Input: part model. Units: mm. Frame: model coordinates. Give positions to 0.01 mm unless a question says otherwise; leave off trailing zeros. Loops run counter-clockwise (first coordinate to the right, second up) from the corner with the lowest first, then second, coordinate; pieces in that order, holes last. Notation, with made-up numbers: (-29.75, 18.25) - (-11.75, 18.25) arc R7 cw to (-11.75, 26.25) - close; hole circle Ø3 at (-4, -11.75). An arc over 180 degrees is marked (long way). One line per item, written item: value.
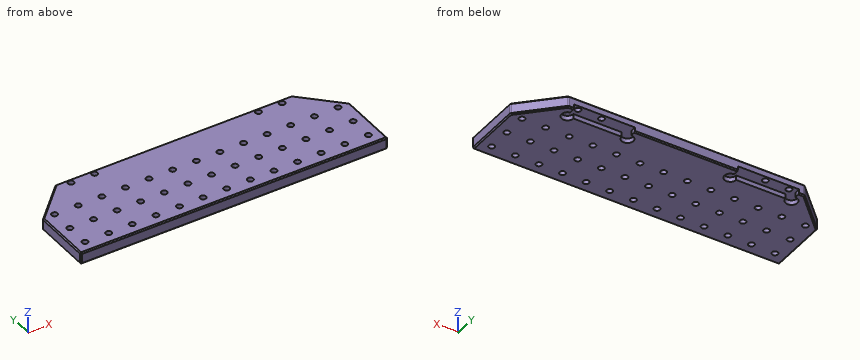
from build123d import *

# Parameters (mm, degrees)
EXTRUDE_1_DEPTH             = 3
EXTRUDE_1_DEPTH_BACK        = 2
SKETCH_2_W                  = 130
SKETCH_2_H                  = 40
SKETCH_6_W                  = 25.903315895
SKETCH_6_H                  = 5
CUT_EXTRUDE_6_DEPTH         = 2
SKETCH_7_R                  = 2.5
CUT_EXTRUDE_7_DEPTH         = 2
CHAMFER_1_SIZE              = 15
M3X0_5_1_D                  = 2.5
M3X0_5_1_DEPTH              = 8.5
M3X0_5_1_TIP                = 0.751075774
FILLET_1_R                  = 1
PATTERN_LINEAR_1_COUNT      = 7
PATTERN_LINEAR_1_PITCH      = 10
PATTERN_LINEAR_1_COUNT_DIR2 = 3
PATTERN_LINEAR_1_PITCH_DIR2 = 10
PATTERN_LINEAR_2_COUNT      = 7
PATTERN_LINEAR_2_PITCH      = 10
PATTERN_LINEAR_2_COUNT_DIR2 = 3
PATTERN_LINEAR_2_PITCH_DIR2 = 10
CHAMFER_2_SIZE              = 0.5


with BuildPart() as part:
    # ｽｹｯﾁ2 → ﾎﾞｽ - 押し出し1 (new, two sides: drawn at the far end of the back side and taken through both)
    with BuildSketch(Plane.XY.offset(-EXTRUDE_1_DEPTH_BACK)):
        with Locations((-80.49999999, -32)):
            Rectangle(SKETCH_2_W, SKETCH_2_H)
    extrude(amount=EXTRUDE_1_DEPTH + EXTRUDE_1_DEPTH_BACK)

    # ｽｹｯﾁ6 → ｶｯﾄ - 押し出し6 (cut)
    with BuildSketch(Plane(origin=(0, 0, -2), x_dir=(-1, 0, 0), z_dir=(0, 0, -1))):
        with Locations((115.230241042, -14.5)):
            Rectangle(SKETCH_6_W, SKETCH_6_H)
        with Locations((45.76975894, -14.5)):
            Rectangle(SKETCH_6_W, SKETCH_6_H)
    extrude(amount=-CUT_EXTRUDE_6_DEPTH, mode=Mode.SUBTRACT)

    # ｽｹｯﾁ7 → ｶｯﾄ - 押し出し7 (cut)
    with BuildSketch(Plane(origin=(0, 0, -2), x_dir=(-1, 0, 0), z_dir=(0, 0, -1))):
        with Locations((33.318100992, -17)):
            Circle(SKETCH_7_R)
        with Locations((128.181898989, -17)):
            Circle(SKETCH_7_R)
        with Locations((102.278583094, -17)):
            Circle(SKETCH_7_R)
        with Locations((58.721416887, -17)):
            Circle(SKETCH_7_R)
    extrude(amount=-CUT_EXTRUDE_7_DEPTH, mode=Mode.SUBTRACT)

    # 面取り1
    chamfer_1_edges = [part.edges().sort_by_distance(p)[0] for p in [
        (-145.49999999, -12, 0.5),
        (-15.49999999, -12, 0.5),
    ]]
    chamfer(chamfer_1_edges, length=CHAMFER_1_SIZE)

    # M3x0.5 ねじ穴1
    with Locations(Plane(origin=(0, 0, 0), x_dir=(-1, 0, 0), z_dir=(0, 0, -1))):
        with Locations((35.818100992, -14), (125.181898989, -14), (45.818100992, -14), (115.181898989, -14)):
            Hole(M3X0_5_1_D / 2, depth=M3X0_5_1_DEPTH)
            with Locations((0, 0, -(M3X0_5_1_DEPTH + M3X0_5_1_TIP / 2))):  # 118° drill point
                Cone(0, M3X0_5_1_D / 2, M3X0_5_1_TIP, mode=Mode.SUBTRACT)

    # ﾌｨﾚｯﾄ1
    fillet_1_edges = [part.edges().sort_by_distance(p)[0] for p in [
        (-30.49999999, -12, 0.5),
        (-130.49999999, -12, 0.5),
        (-145.49999999, -27, 0.5),
        (-15.49999999, -27, 0.5),
    ]]
    fillet(fillet_1_edges, radius=FILLET_1_R)

    # ｽｹｯﾁ11 → M3x0.5 ねじ穴2 (revolve, cut)
    with BuildSketch(Plane(origin=(-80.49999999, -47, -2), x_dir=(0, 1, 0), z_dir=(1, 0, 0))):
        Polygon((0, 0), (0, 9.251075774), (1.25, 8.5), (1.25, 0), align=None)
    m3x0_5_2 = revolve(axis=Axis((-80.49999999, -47, -8.35), (0, 0, 1)), mode=Mode.SUBTRACT)

    # 直線ﾊﾟﾀｰﾝ1: M3x0.5 _2 7 × 3
    with Locations(*[(i * PATTERN_LINEAR_1_PITCH, j * PATTERN_LINEAR_1_PITCH_DIR2, 0) for i in range(PATTERN_LINEAR_1_COUNT) for j in range(PATTERN_LINEAR_1_COUNT_DIR2) if (i, j) != (0, 0)]):
        add(m3x0_5_2, mode=Mode.SUBTRACT)

    # 直線ﾊﾟﾀｰﾝ2: M3x0.5 _2 7 × 3
    with Locations(*[(-i * PATTERN_LINEAR_2_PITCH, j * PATTERN_LINEAR_2_PITCH_DIR2, 0) for i in range(PATTERN_LINEAR_2_COUNT) for j in range(PATTERN_LINEAR_2_COUNT_DIR2) if (i, j) != (0, 0)]):
        add(m3x0_5_2, mode=Mode.SUBTRACT)

    # 面取り2
    chamfer_2_edges = [part.edges().sort_by_distance(p)[0] for p in [
        (-15.49999999, -39.707106781, -2),
        (-80.49999999, -52, 3),
        (-15.49999999, -39.707106781, 3),
        (-145.49999999, -39.707106781, 3),
        (-145.49999999, -39.707106781, -2),
        (-137.99999999, -19.5, -2),
        (-31.866157273, -12, -2),
        (-22.99999999, -19.5, -2),
        (-15.576120458, -27.03153013, -2),
        (-30.53153012, -12.076120467, -2),
        (-130.46846986, -12.076120467, -2),
        (-145.423879523, -27.03153013, -2),
        (-137.99999999, -19.5, 3),
        (-80.49999999, -12, 3),
        (-22.99999999, -19.5, 3),
        (-15.576120458, -27.03153013, 3),
        (-30.53153012, -12.076120467, 3),
        (-130.46846986, -12.076120467, 3),
        (-145.423879523, -27.03153013, 3),
        (-80.49999999, -12, -2),
        (-129.133842708, -12, -2),
        (-80.49999999, -52, -2),
        (-15.49999999, -52, 0.5),
        (-145.49999999, -52, 0.5),
    ]]
    chamfer(chamfer_2_edges, length=CHAMFER_2_SIZE)


solid = part.part
Item 1: Material intervals for L1, parallel to Z at x = -120.5, y = -14; L2, parallel to Y at x = -100, z = 0.55; L3, parallel to X at y = -13.5, z = -1.1, sorted ascending.
Verdict:
L1: z = 0 to 3
L2: y = -52 to -48.15, -45.85 to -38.15, -35.85 to -28.15, -25.85 to -12
L3: x = -132 to -128.18, -102.28 to -58.72, -32.82 to -29
Item 2: Pin query (flat end, axial travel): P1, Ø2, axis at x = -59.5, y = -27.5, coming from the -Z side; P2, Ø3, axis at x = -102.28, y = -17, coming from the -Z side; P3, Ø1.5, axis at y = -26.5, z = -1, coming from the +X side; P4, Ø0.6, axis at x = -113.5, z = -1.5, coming from the +Y side. Return the tip coordinate at first contact, or that it passes through.
Verdict:
P1: stops at z = -2
P2: stops at z = 0
P3: stops at x = -15.51
P4: stops at y = -17
Item 3: Section B-B, the plane x = -50.5. Output: boundary loops of the cut face in (y, z), and give its area (3 significant figures).
Verdict:
outline: (-52, -1.5) - (-51.5, -2) - (-48.25, -2) - (-48.25, 3) - (-51.5, 3) - (-52, 2.5) - close; (-45.75, -2) - (-38.25, -2) - (-38.25, 3) - (-45.75, 3) - close; (-35.75, -2) - (-28.25, -2) - (-28.25, 3) - (-35.75, 3) - close; (-25.75, -2) - (-17, -2) - (-17, 0) - (-12, 0) - (-12, 2.5) - (-12.5, 3) - (-25.75, 3) - close
area: 152 mm^2
Item 4: Section A-A, the plane x = -70.5. Output: boundary loops of the cut face in (y, z), and give its area (3 significant figures).
Verdict:
outline: (-52, -1.5) - (-51.5, -2) - (-48.25, -2) - (-48.25, 3) - (-51.5, 3) - (-52, 2.5) - close; (-45.75, -2) - (-38.25, -2) - (-38.25, 3) - (-45.75, 3) - close; (-35.75, -2) - (-28.25, -2) - (-28.25, 3) - (-35.75, 3) - close; (-25.75, -2) - (-12.5, -2) - (-12, -1.5) - (-12, 2.5) - (-12.5, 3) - (-25.75, 3) - close
area: 162 mm^2
Item 5: Section D-D, the plane y = -24. Output: boundary loops of the cut face in (x, z).
Verdict:
outline: (-142.5, -1.5) - (-141.79, -2) - (-19.21, -2) - (-18.5, -1.5) - (-18.5, 2.5) - (-19.21, 3) - (-141.79, 3) - (-142.5, 2.5) - close
Item 6: Section C-C, the plane y = -37. Count the separate pieces of the cut face and the enclosed holes in it, and give its area (3 significant figures).
Verdict:
separate pieces: 14
enclosed holes: 0
area: 487 mm^2
